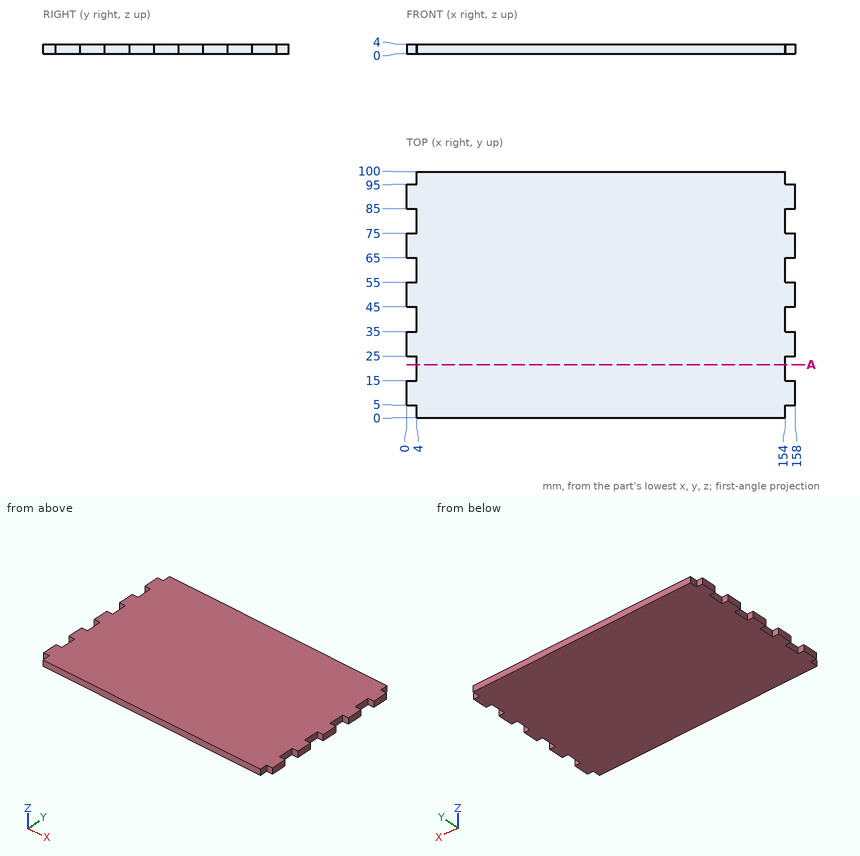
Job drawing, mm, ordinate dimensions from the low corner. One solid piece. Give positions to 0.01 mm unless a question says otherwise; leave off trailing zeros. Loops run counter-clockwise (first coordinate to the right, second up) from the corner with the lowest first, then second, coordinate; pieces in that order, holes last. Notation, with made-up numbers: M 0,21 L 52,21 A18 ccw 52,45 Z; hole C -3.75,44 d8. An arc over 180 degrees is marked long. Use one line per item in the form item = value.
Item 1: Flat gauge pins, fed straight in: pin 1 Ø2 at (x, z) = (156.5, 2.5) entering from -Y; pin 2 Ø2 at (y, z) = (62, 1) entering from -X; pin 3 Ø1.2 at (x, z) = (156.5, 1) entering from +Y. Where does each tip first touch, or does it go through?
Filled in:
pin_1 = 5
pin_2 = 4
pin_3 = 95
Item 2: Drill centre line: L1, parallel to X at y = 56.5, z = 1.2. Where is it in solid material? Low to high.
Filled in:
L1 = 4 to 154
Item 3: Slice it at A-A on y = 21.5. List the corners of the cut face in (x, z).
Filled in:
outline = M 4,0 L 154,0 L 154,4 L 4,4 Z
